Build history of the part. All positions in model axes, mm. A direction names the side the tool comes from. Round coordinates to 2 decimals unless told otherwise and drop trailing zeros. Loops run counter-clockwise (first coordinate to the right, second up) from the corner with the lowest first, then second, coordinate; pieces in that order, holes last. Notation, with made-up numbers: (17.5, 74.5) -> (39.5, 74.5) arc R11 ccw to (39.5, 86.5) -> close; hole circle Ø5 at (-35.75, 78). An arc over 180 degrees is marked (long way). Put each result on its own line as item: value. Start each with the question number.
Item 1: Cut at C-C, the plane z = 1.75. List the corners of the cut face in (x, y).
Item 2: Tool access for faces 5 (the flat face through (12, 96, 0)), 6 (the flat face through (25, 96, 2)): list every direction of +Z, -Z, +X, -X, +Y, -Y with a clear straight run to the whole face (end or side of a thin tool).
Item 3: Cut at D-D, the plane y = 23.5. List the corners of the cut face in (x, z).
Item 4: Flat gauge pins, fed straight in: pin 1 Ø5 at (x, y) = (18.25, 15) entering from -Z; pin 2 Ø12.5 at (x, y) = (13, 88.5) entering from -Z; pin 3 Ø10 at (y, z) = (120, -12.5) entering from +X. Where does each tip first touch, or does it go through?
Item 5: Cut at A-A, the plane x = 18.25. List the corners of the cut face in (y, z), plus the area to 3 significant figures.
Item 6: Pull direction Y, two halves, no side cores. Call faces 1 (the cylindrical face through (17.697, 184.214, 2.028)), 2 (the flat face through (4, 0, 1)), 3 (the cylindrical face through (20.21, 93.73, 2.03)), 4 (the flat face through (0, 99, -11)): +Y half, -Y half, draft (parallel to the pull), parting line (faces both ways), or undercut.
Item 7: Drill centre lines: probe 1 along Y at (x, z) = (18.25, 3.15); probe 2 along Z at (x, y) = (2.75, 36); probe 3 along X at (y, z) = (163, -10). Where is each one in solid material? Low to high. Write a range as [from, to].
Item 8: Cut at B-B, the plane y = 180. List the corners of the cut face in (x, z), plus the area to 3 significant figures.
```python
from build123d import *

# Parameters (mm, degrees)
CROQUIS1_W              = 25
CROQUIS1_H              = 3
SALIENTE_EXTRUIR1_DEPTH = 195
CROQUIS2_R              = 4.25
CORTAR_EXTRUIR1_DEPTH   = 195
CROQUIS3_W              = 4
CROQUIS3_H              = 25
SALIENTE_EXTRUIR2_DEPTH = 195
SALIENTE_EXTRUIR3_START = 1
CROQUIS4_W              = 29
CROQUIS4_H              = 195
CROQUIS4_R              = 4.25
SALIENTE_EXTRUIR3_DEPTH = 1


with BuildPart() as part:
    # Croquis1 → Saliente-Extruir1 (new body)
    with BuildSketch(Plane(origin=(0, 0, 0), x_dir=(1, 0, 0), z_dir=(0, 1, 0))):
        with Locations((12.5, -1.5)):
            Rectangle(CROQUIS1_W, CROQUIS1_H)
    extrude(amount=SALIENTE_EXTRUIR1_DEPTH)

    # Croquis2 → Cortar-Extruir1 (cut)
    with BuildSketch(Plane.XY.offset(3)):
        with Locations((18.25, 180)):
            Circle(CROQUIS2_R)
        with Locations((18.25, 97.5)):
            Circle(CROQUIS2_R)
        with Locations((18.25, 15)):
            Circle(CROQUIS2_R)
    extrude(amount=-CORTAR_EXTRUIR1_DEPTH, mode=Mode.SUBTRACT)

    # Croquis3 → Saliente-Extruir2 (add)
    with BuildSketch(Plane(origin=(0, 195, 0), x_dir=(1, 0, 0), z_dir=(0, 1, 0))):
        with Locations((-2, 9.5)):
            Rectangle(CROQUIS3_W, CROQUIS3_H)
    extrude(amount=-SALIENTE_EXTRUIR2_DEPTH)

    # Croquis4 → Saliente-Extruir3 (add)
    with BuildSketch(Plane.XY.offset(3).offset(SALIENTE_EXTRUIR3_START)):
        with Locations((10.5, 97.5)):
            Rectangle(CROQUIS4_W, CROQUIS4_H)
        with Locations((18.25, 15)):
            Circle(CROQUIS4_R, mode=Mode.SUBTRACT)
        with Locations((18.25, 97.5)):
            Circle(CROQUIS4_R, mode=Mode.SUBTRACT)
        with Locations((18.25, 180)):
            Circle(CROQUIS4_R, mode=Mode.SUBTRACT)
    extrude(amount=-SALIENTE_EXTRUIR3_DEPTH)


solid = part.part
```
Reply:
1. outline: (-4, 0) -> (25, 0) -> (25, 195) -> (-4, 195) -> close; hole circle Ø8.5 at (18.25, 15); hole circle Ø8.5 at (18.25, 97.5); hole circle Ø8.5 at (18.25, 180)
2. face 5: -Z, +X, +Y, -Y
2. face 6: +Z, -Z, +X, +Y, -Y
3. outline: (-4, -22) -> (0, -22) -> (0, 0) -> (25, 0) -> (25, 4) -> (-4, 4) -> close
4. pin 1: passes through
4. pin 2: stops at z = 0
4. pin 3: stops at x = 0
5. outline: (0, 0) -> (10.75, 0) -> (10.75, 4) -> (0, 4) -> close; (19.25, 0) -> (93.25, 0) -> (93.25, 4) -> (19.25, 4) -> close; (101.75, 0) -> (175.75, 0) -> (175.75, 4) -> (101.75, 4) -> close; (184.25, 0) -> (195, 0) -> (195, 4) -> (184.25, 4) -> close
5. area: 678 mm^2
6. face 1: undercut
6. face 2: -Y half
6. face 3: undercut
6. face 4: draft
7. probe 1: y = [0, 10.75], [19.25, 93.25], [101.75, 175.75], [184.25, 195]
7. probe 2: z = [0, 4]
7. probe 3: x = [-4, 0]
8. outline: (-4, -22) -> (0, -22) -> (0, 0) -> (14, 0) -> (14, 4) -> (-4, 4) -> close; (22.5, 0) -> (25, 0) -> (25, 4) -> (22.5, 4) -> close
8. area: 170 mm^2
